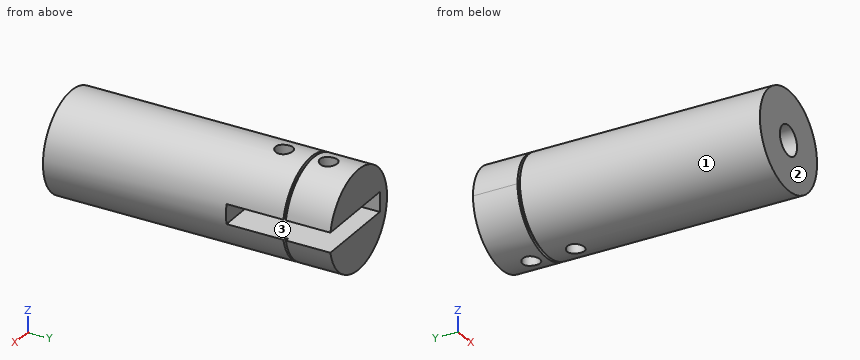
Autodesk Inventor part; units mm, degrees
ref_plane "TopGroovePlane" through (-7.5, -3, -2) normal (0, 1, 0) x (1, 0, 0)
ref_plane "YZ Plane" through (0, 0, 0) normal (1, 0, 0) x (0, 1, 0)
ref_plane "XZ Plane" through (0, 0, 0) normal (0, 1, 0) x (-1, 0, 0)
sketch "Body" plane through (0, 0, 0) normal (0, 0, 1) x (1, 0, 0)
  circle A0 centre (0, 0) radius 1.75
  line L0 (-10, -52) -> (10, -52)
  line L1 (10, 6) -> (-10, 6)
  line L2 (10, 6) -> (10, -52)
  line L3 (-10, 6) -> (-10, -52)
  line L4 (0, -52) -> (0, 6)
  line L5 (10, -15) -> (-10, -15)
  circle A1 centre (0, -9) radius 1.75
  circle A2 centre (0, 0) radius 2.75 construction
  circle A3 centre (0, -9) radius 2.75 construction
  line L6 (-7.5, 6) -> (-7.5, -15)
  dimension "d0" = 58
  dimension "d2" = 3.5
  dimension "d3" = 6
  dimension "d5" = 10
  dimension "d6" = 20
  dimension "d7" = 9
  dimension "d23" = 5.5
  dimension "d25" = 6
  dimension "d26" = 2.5
revolve "BodyFeature" add sketch "Body" angle 360 about axis through (0, -52, 0) along (0, 1, 0) picked at (-0.4801, -0.3314) picked at (-0.4801, -8.6686) contours L4 A0 | A0 L4 A1 L5 L6 L1 | L4 A1 | L6 L5 L3 L1 | L5 L4 L0 L3
extrude "HolesFeature" cut sketch "Body" along normal through all both and the other way through all contours A0 L4 | L4 A0 | A1 L4 | L4 A1
extrude "MountFeature" cut sketch "Body" along normal mid plane 4 contours A0 L4 L1 L2 L5 A1 | A0 L4 A1 L5 L6 L1
ref_plane "TopGroovePlane" through (-7.5, -3, -2) normal (0, 1, 0) x (1, 0, 0)
sketch "TopGroove" plane through (-7.5, -3, -2) normal (0, 1, 0) x (1, 0, 0)
  circle A0 centre (7.5, -2) radius 10
  circle A1 centre (7.5, -2) radius 9.3
  dimension "d30" = 0.7
extrude "TopGrooveFeature" cut sketch "TopGroove" against normal blind 0.5
sketch "BottomMountHole" plane through (0, -52, 0) normal (0, -1, 0) x (1, 0, 0)
  circle A0 centre (0, 0) radius 10
hole "BottomMountHoleFeature" at (0, -52, 0) direction (0, 1, 0) diameter 6 depth 30 tip angle 118
properties part number "PelvisMountStem"
Model file for the job. Use its own axes, mm. Face numbers are marked on the shaded views. Give positions to 0.01 mm unless a question says otherwise; leave off trailing zeros. Loops run counter-clockwise (first coordinate to the right, second up) from the corner with the lowest first, then second, coordinate; pieces in that order, holes last.
1) Saw through at A-A (y = -36). Write the cut outline in (x, z).
2) Saw through at D-D (x = -6). Write the cut outline in (y, z), plus the area to 3 significant figures.
3) Saw through at B-B (z = -5.5). Write the cut outline in (x, y).
4) Flat gauge pins, fed straight in: pin 1 Ø1 at (x, y) = (3.5, -3.5) entering from +Z; pin 2 Ø5 at (x, y) = (4, -3.5) entering from -Z; pin 3 Ø2 at (x, y) = (0, 0) entering from +Z; pin 4 Ø6 at (x, y) = (-7, -12) entering from -Z. Where does each tip first touch, or does it go through?
5) Pull direction Z, two halves, no side cores. Call the marked faces 1, 2 and 3: +Z half, -Z half, draft (parallel to the pull), parting line (faces both ways), or undercut.
6) Wall check: line 1 (Y direction, x = 0, z = -4); line 2 (Z direction, x = -0.25, y = -26); line 3 (X direction, y = -33, z = 0). Give the ranges that are in metal, low to high.
7) Saw through at C-C (y = 0). Write the cut outline in (x, z), plus the area to 3 significant figures.
Answer block:
1. outline: circle Ø20 at (0, 0); hole circle Ø6 at (0, 0)
2. outline: (-52, -8) - (-3.5, -8) - (-3.5, -7.11) - (-3, -7.11) - (-3, -8) - (6, -8) - (6, -2) - (-15, -2) - (-15, 2) - (6, 2) - (6, 8) - (-3, 8) - (-3, 7.11) - (-3.5, 7.11) - (-3.5, 8) - (-52, 8) - close
2. area: 843 mm2
3. outline: (-8.35, -52) - (8.35, -52) - (8.35, -3.5) - (7.5, -3.5) - (7.5, -3) - (8.35, -3) - (8.35, 6) - (-8.35, 6) - (-8.35, -3) - (-7.5, -3) - (-7.5, -3.5) - (-8.35, -3.5) - close; hole circle Ø3.5 at (0, -9); hole circle Ø3.5 at (0, 0)
4. pin 1: stops at z = 9.54
4. pin 2: stops at z = -9.89
4. pin 3: passes through
4. pin 4: stops at z = -9.17
5. face 1: parting line
5. face 2: draft
5. face 3: undercut
6. line 1: y = -52 to -10.75, -7.25 to -1.75, 1.75 to 6
6. line 2: z = -10 to -2.99, 2.99 to 10
6. line 3: x = -10 to -3, 3 to 10
7. outline: (-7.5, -2) - (-7.5, 2) - (-1.75, 2) - (-1.75, 9.85) arc R10 ccw to (-1.75, -9.85) - (-1.75, -2) - close; (1.75, -9.85) arc R10 ccw to (9.8, -2) - (1.75, -2) - close; (1.75, 2) - (9.8, 2) arc R10 ccw to (1.75, 9.85) - close
7. area: 189 mm2
